from build123d import *

# Parameters (mm, degrees)
SKETCH_1_W      = 10
SKETCH_1_H      = 3.1
EXTRUDE_1_DEPTH = 3.1
SKETCH_2_W      = 20
SKETCH_2_H      = 25
EXTRUDE_2_DEPTH = 3.1


with BuildPart() as part:
    # 草图1 → 凸台-拉伸1 (new body)
    with BuildSketch(Plane(origin=(0, 0, 0), x_dir=(1, 0, 0), z_dir=(0, 1, 0))):
        Polygon((-35, 50), (-35, -50), (-14.875, -50), (-4.875, -50), (-1.5, -50), (-1.5, -47), (-3.25, -47), (-3.25, -44.45), (-1.5, -44.45), (-1.5, -40.1), (1.5, -40.1), (1.5, -44.45), (3.25, -44.45), (3.25, -47), (1.5, -47), (1.5, -50), (4.875, -50), (14.875, -50), (35, -50), (35, 50), (14.875, 50), (4.875, 50), (1.5, 50), (1.5, 47), (3.25, 47), (3.25, 44.45), (1.5, 44.45), (1.5, 40.1), (-1.5, 40.1), (-1.5, 44.45), (-3.25, 44.45), (-3.25, 47), (-1.5, 47), (-1.5, 50), (-4.875, 50), (-14.875, 50), align=None)
        with Locations((-9.875, 51.55)):
            Rectangle(SKETCH_1_W, SKETCH_1_H)
        with Locations((9.875, 51.55)):
            Rectangle(SKETCH_1_W, SKETCH_1_H)
        with Locations((-9.875, -51.55)):
            Rectangle(SKETCH_1_W, SKETCH_1_H)
        with Locations((9.875, -51.55)):
            Rectangle(SKETCH_1_W, SKETCH_1_H)
    extrude(amount=EXTRUDE_1_DEPTH)

    # 草图2 → 凸台-拉伸2 (add)
    with BuildSketch(Plane(origin=(0, 0, 0), x_dir=(1, 0, 0), z_dir=(0, 1, 0))):
        with Locations((45, 37.5)):
            Rectangle(SKETCH_2_W, SKETCH_2_H)
        with Locations((45, -37.5)):
            Rectangle(SKETCH_2_W, SKETCH_2_H)
    extrude(amount=EXTRUDE_2_DEPTH)


solid = part.part
Input: part model. Units: mm. Frame: model coordinates. A direction names the side the tool comes from. Give positions to 0.01 mm unless a question says otherwise; leave off trailing zeros. Order: outer loops, then holes, each group sorted by start corner. A loop starts at its lowest first (then second) coordinate and runs counter-clockwise, first axis right, second up. Notation, with made-up numbers: (-1.5, -22) - (37.5, -22) arc R22 cw to (37.5, 4) - close; hole circle Ø8 at (85, 42). An arc over 180 degrees is marked (long way). Answer as a JSON object with one key per item and string values. Group by question number.
Q1. Cut plane B-B, the plane z = 7.5. Output: boundary loops of the cut face in (x, y).
Q2. Cut plane C-C, the plane x = 21.5. Output: boundary loops of the cut face in (y, z), then the cut area to 3 significant figures.
Q3. Mould query, pull axis Z, two halves, no side actions, for faces 6 (the face through (-14.875, 2, -52)), 7 (the face through (45, 2, -25)), 8 (the face through (-25, 2, 50)). Classes: pulls with the +Z half, pulls with the -Z half, needs draft (parallel to the pull), parting line crosses it, or undercut.
Q4. Line query: probe 1 along Z at (x, y) = (-2.5, 0.95); probe 2 along Z at (x, y) = (46, 1.35); probe 3 along X at (y, z) = (1.05, -2). Output: solid intervals per line, ascending.
Q5. Cut plane A-A, the plane x = 37.5. Output: boundary loops of the cut face in (y, z).
Q6. Set-up query: faces 1 (the face through (3.25, 2, 46)), 2 (the face through (-25, 2, -50)), 3 (the face through (35, 2, -50)), 4 (the face through (-1.5, 2, -42)), 5 (the face through (45, 2, 25)). Return all of +Z, -Z, +X, -X, +Y, -Y with unobstructed straight access to the full face (end or side cutting, diameter ignored); none if empty.
Q7. First-contact query: pin 1 Ø0.5 at (x, y) = (-2.5, 2.5) entering from +Z; pin 2 Ø0.5 at (x, y) = (2, 1) entering from -Z. Flat tips, straight axial feed; report the tip coordinate or a pass-through.
Results:
{
 "1": {"outline": "(-35, 0) - (35, 0) - (35, 3.1) - (-35, 3.1) - close"},
 "2": {"outline": "(0, -50) - (3.1, -50) - (3.1, 50) - (0, 50) - close", "area": "310 mm^2"},
 "3": {"face 6": "needs draft", "face 7": "undercut", "face 8": "pulls with the +Z half"},
 "4": {"probe 1": "-50 to -47, -44.45 to 44.45, 47 to 50", "probe 2": "-50 to -25, 25 to 50", "probe 3": "-35 to 35"},
 "5": {"outline": "(0, -50) - (3.1, -50) - (3.1, -25) - (0, -25) - close; (0, 25) - (3.1, 25) - (3.1, 50) - (0, 50) - close"},
 "6": {"face 1": "+Y, -Y", "face 2": "-Z, -X, +Y, -Y", "face 3": "-Z, +X, +Y, -Y", "face 4": "-Z, +Y, -Y", "face 5": "+X, +Y, -Y"},
 "7": {"pin 1": "z = 50", "pin 2": "z = -50"}
}
